Input: dimensioned drawing with shaded views. Units: mm. Origin: part minimum x, y, z. A direction names the side the tool comes from. Coordinates: 2 decimals unless noted, no trailing zeros. Order: outer loops, then holes, each group sorted by start corner. A loop starts at its lowest first (then second) coordinate and runs counter-clockwise, first axis right, second up. Notation, with made-up numbers: (1, 73) -> (43, 73) arc R25 ccw to (43, 90) -> close; hole circle Ø1 at (20.5, -20.75). An arc over 180 degrees is marked (long way). Answer in a Markdown table with one row per item. Add a question column.
1) Contact query for flat-ended pins moving along their axis: P1, Ø3, axis at y = 28.5, z = 18.5, coming from the +X side; P2, Ø1.5, axis at x = 94, y = 50.5, coming from the -Z side; P3, Ø2, axis at y = 14.5, z = 11.5, coming from the -X side; P4, Ø1, axis at y = 47.5, z = 49.5, coming from the -X side. Output: stop coordinate, or through.
2) Section query C-C on x = 86. Return the cut outline in (y, z).
3) Section query D-D on y = 5.5. Return the cut outline in (x, z), then the cut area to 3 significant figures.
4) Ray query, line 1 (Z direction, x = 140, y = 40); line 2 (X direction, y = 65.5, z = 23). Return the intervals inside material, ascending. Write a range as from..to.
5) Set-up query: the marked faces 1, 2 and 3. Return all of +Z, -Z, +X, -X, +Y, -Y with unobstructed straight access to the full face (end or side cutting, diameter ignored); none if empty.
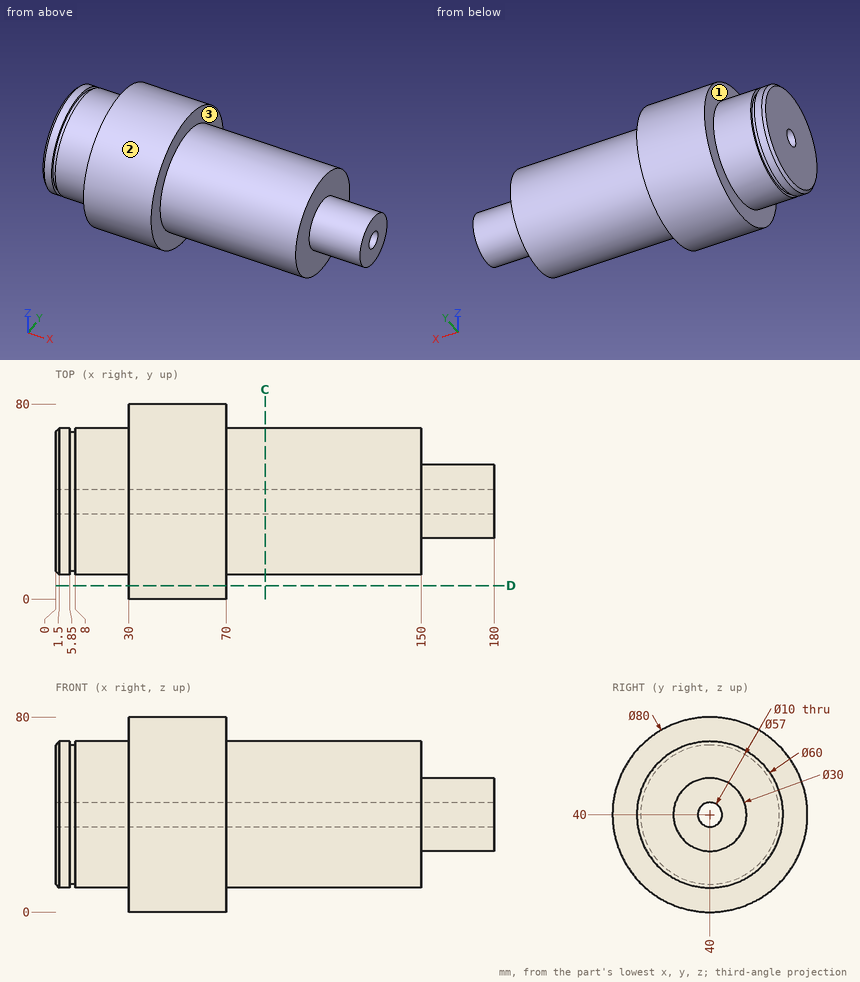
Result:
| question | item | result |
|---|---|---|
| 1 | P1 | x = 150 |
| 1 | P2 | z = 11.63 |
| 1 | P3 | x = 30 |
| 1 | P4 | x = 0 |
| 2 | outline | circle Ø60 at (40, 40); hole circle Ø10 at (40, 40) |
| 3 | outline | (30, 19.76) -> (70, 19.76) -> (70, 60.24) -> (30, 60.24) -> close |
| 3 | area | 1,620 mm2 |
| 4 | line 1 | 10..35, 45..70 |
| 4 | line 2 | 30..70 |
| 5 | face 1 | -X |
| 5 | face 2 | +X, -X |
| 5 | face 3 | +X |
